from build123d import *

# Parameters (mm, degrees)
F0_W     = 20
F0_H     = 20
F1_DEPTH = 5
F2_T     = -0.5
F3_W     = 20
F3_H     = 20
F4_DEPTH = 1.2


with BuildPart() as f1:
    # F0 (on Top) → F1 (new body)
    with BuildSketch(Plane.XY):
        Rectangle(F0_W, F0_H)
    extrude(amount=F1_DEPTH)

    # F2
    f2_openings = [f1.faces().sort_by_distance(p)[0] for p in [
        (0, 0, 5),
        (0, 0, 0),
    ]]
    offset(amount=F2_T, openings=f2_openings)

    # F3 (on Top) → F4 (join)
    with BuildSketch(Plane.XY):
        Rectangle(F3_W, F3_H)
    extrude(amount=F4_DEPTH)


solid = f1.part
Geometry check sheet. Reference: the model listing, model coordinates, mm. A direction names the side the tool comes from. Coordinates: 2 decimals unless noted, no trailing zeros. Order: outer loops, then holes, each group sorted by start corner. A loop starts at its lowest first (then second) coordinate and runs counter-clockwise, first axis right, second up. Notation, with made-up numbers: (26, 46.5) -> (61, 46.5) arc R24 ccw to (61, 85.5) -> close; hole circle Ø8 at (42, 87.25). An arc over 180 degrees is marked (long way). Use a Markdown table: item, result. Add a question column.
1. Cross-section at B-B (x = 2.25). Enter the section's corners in (y, z), and give its area (3 significant figures).
2. Material ranges on L1, parallel to Y at x = 7.5, z = 4.55; L2, parallel to Z at x = -3.5, y = -2, recorded low to high.
3. Set-up check for faces 4 (the face through (-9.5, 0, 3)), 5 (the face through (0, 0, 0)): record each of +Z, -Z, +X, -X, +Y, -Y from which the full face is reachable in a straight line by a thin tool's end or side.
4. Go/stop test with a flat-tipped pin: pin 1 Ø2 at (x, y) = (-2.5, -4.5) entering from +Z. Record where the tip stops, or that it passes through.
5. Mould release check, pull along Y, two halves, no side actions. Record for faces 1 (the face through (10, 0, 2)), 2 (the face through (0, -10, 2)), 3 (the face through (9.5, 0, 3)): pulls with the +Y half, pulls with the -Y half, needs draft (parallel to the pull), parting line crosses it, or undercut.
6. Cross-section at A-A (z = 2.5). Enter the section's corners in (x, y).
Filled sheet:
| question | item | result |
|---|---|---|
| 1 | outline | (-10, 0) -> (10, 0) -> (10, 5) -> (9.5, 5) -> (9.5, 1.2) -> (-9.5, 1.2) -> (-9.5, 5) -> (-10, 5) -> close |
| 1 | area | 27.8 mm2 |
| 2 | L1 | -10 to -9.5, 9.5 to 10 |
| 2 | L2 | 0 to 1.2 |
| 3 | face 4 | +Z |
| 3 | face 5 | -Z, +X, -X, +Y, -Y |
| 4 | pin 1 | z = 1.2 |
| 5 | face 1 | needs draft |
| 5 | face 2 | pulls with the -Y half |
| 5 | face 3 | undercut |
| 6 | outline | (-10, -10) -> (10, -10) -> (10, 10) -> (-10, 10) -> close; hole (-9.5, -9.5) -> (9.5, -9.5) -> (9.5, 9.5) -> (-9.5, 9.5) -> close |
